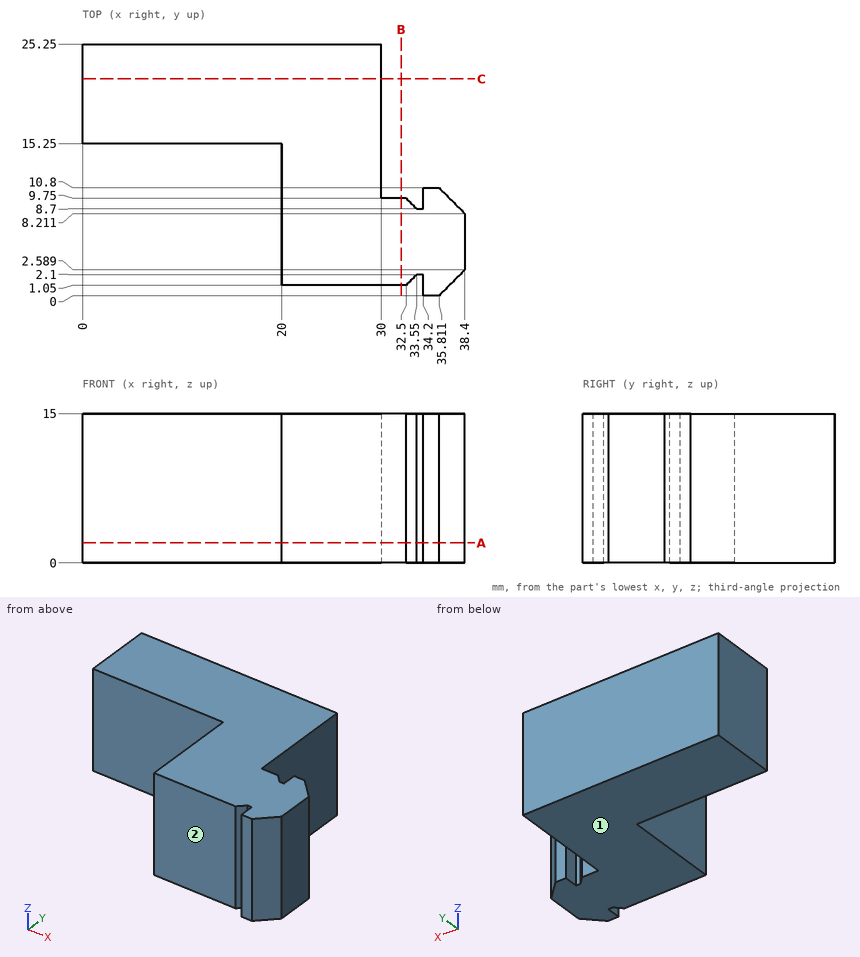
Design review of the part shown in the three views and the two pictorial views. Dimensions are in mm from the part's minimum x, y and z. A direction names the side the tool comes from. Give positions to 0.01 mm unless a question says otherwise; leave off trailing zeros. Write each loop counter-clockwise with the first axis right and the second up, starting at its lowest first coordinate (ties: lowest second). Pieces come first, ordered by that corner, then holes.
Item 1: Machinability: for the marked faces 1 and 2, which of the approach directions +Z, -Z, +X, -X, +Y, -Y give a long, thin tool a straight path to every point of the face, cutting with its end or side? Answer none if there is none.
Item 2: Take a section at A-A (z = 2). Give the boundary of the cut face in (x, y).
Item 3: Wall thickness on probe 1 along Y at (x, z) = (5.5, 4.25); probe 2 along X at (y, z) = (22.75, 10); probe 3 along X at (y, z) = (13.5, 7.25): over which ranges is each line inside the solid? List them lowest first.
Item 4: Insertion check: P1, Ø4.5, axis at y = 18, z = 11, coming from the +X side; P2, Ø0.6, axis at y = 1.5, z = 6, coming from the -X side; P3, Ø1, axis at x = 9, z = 1.5, coming from the -Y side. Each pin has a flat end and moves straight along its axis. Give the tip position at first contact, or say it passes through.
Item 5: Take a section at B-B (x = 32). Give the boundary of the cut face in (y, z), and give its area (4 significant figures).
Item 6: Take a section at C-C (y = 21.75). Give the boundary of the cut face in (x, z), and give its area (3 significant figures).
Established:
1. face 1: -Z, +X, -X, +Y, -Y
1. face 2: +Z, -Z, -X, -Y
2. outline: (0, 15.25) - (20, 15.25) - (20, 1.05) - (32.5, 1.05) - (33.55, 2.1) - (34.2, 2.1) - (34.2, 0) - (35.81, 0) - (38.4, 2.59) - (38.4, 8.21) - (35.81, 10.8) - (34.2, 10.8) - (34.2, 8.7) - (33.55, 8.7) - (32.5, 9.75) - (30, 9.75) - (30, 25.25) - (0, 25.25) - close
3. probe 1: y = 15.25 to 25.25
3. probe 2: x = 0 to 30
3. probe 3: x = 20 to 30
4. P1: stops at x = 30
4. P2: stops at x = 20
4. P3: stops at y = 15.25
5. outline: (1.05, 0) - (9.75, 0) - (9.75, 15) - (1.05, 15) - close
5. area: 130.5 mm2
6. outline: (0, 0) - (30, 0) - (30, 15) - (0, 15) - close
6. area: 450 mm2
